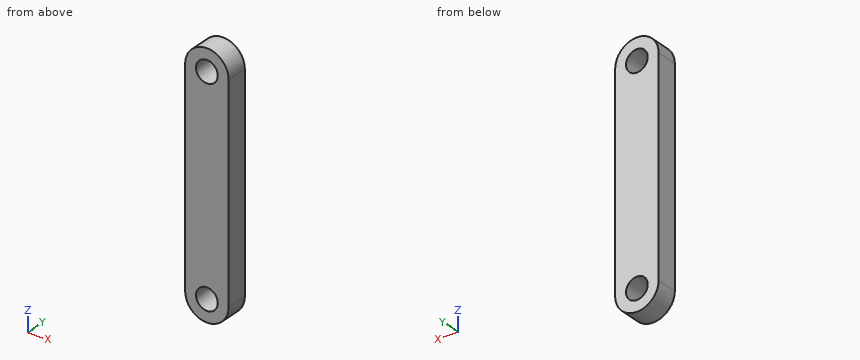
Autodesk Inventor part; units mm, degrees
ref_plane "YZ Plane" through (0, 0, 0) normal (1, 0, 0) x (0, 1, 0)
ref_plane "XZ Plane" through (0, 0, 0) normal (0, 1, 0) x (-1, 0, 0)
ref_plane "XY Plane" through (0, 0, 0) normal (0, 0, 1) x (1, 0, 0)
sketch "Boceto1" plane through (0, 0, 0) normal (0, 1, 0) x (-1, 0, 0)
  line L0 (0, -14.5) -> (0, 14.5) construction
  line L1 (3, -14.5) -> (3, 14.5)
  line L2 (-3, 14.5) -> (-3, -14.5)
  arc A0 (-3, -14.5) -> (3, -14.5) centre (0, -14.5) ccw
  arc A1 (3, 14.5) -> (-3, 14.5) centre (0, 14.5) ccw
  point P0 (0, 0)
  point P1 (0, 17.5)
  point P2 (0, -17.5)
  dimension "d0" = 14.5
  dimension "d1" = 6
extrude "Extrusión1" add sketch "Boceto1" along normal mid plane 3
sketch "Boceto2" plane through (0, 1.5, 0) normal (0, 1, 0) x (1, 0, 0)
  arc A0 (-3, -14.5) -> (3, -14.5) centre (0, -14.5) ccw construction
  arc A1 (3, 14.5) -> (-3, 14.5) centre (0, 14.5) ccw construction
  circle A2 centre (0, -14.5) radius 1.5
  circle A3 centre (0, 14.5) radius 1.5
  point P0 (0, 0)
  dimension "d4" = 3
  dimension "d5" = 3
extrude "Extrusión2" cut sketch "Boceto2" against normal blind 3
equation "\"Radio_pliegue\" = Grosor"
equation "\"Anchura_desahogo_plegado\" = Grosor"
equation "\"Profundidad_desahogo_plegado\" = 0.5 * Grosor"
equation "\"Tamaño_destalonado\" = 4 * Grosor"
equation "\"Remanente_mínimo\" = 2 * Grosor"
equation "\"Radiodetransición\" = Radio_pliegue"
equation "\"Tamaño_de_radio_de_Jacobi\" = Radio_pliegue"
equation "\"TamañoSeparación\" = Grosor"
properties part number "Pinza_pieza2"
Geometry: final body of the model. Coordinates: model frame, mm. Coordinates: 2 decimals unless noted, no trailing zeros. Order: outer loops, then holes, each group sorted by start corner. A loop starts at its lowest first (then second) coordinate and runs counter-clockwise, first axis right, second up. Notation, with made-up numbers: (56, -8.75) -> (94, -8.75) arc R21 cw to (94, -4.75) -> close; hole circle Ø5 at (21.5, 56.5). An arc over 180 degrees is marked (long way). Write each question's results on one line, items separated by ' | '. Start each with the question number.
1) Cut plane B-B, the plane y = 0.1. Output: boundary loops of the cut face in (x, z).
2) Cut plane C-C, the plane z = 15. Output: boundary loops of the cut face in (x, y), and give its area (3 significant figures).
3) Material intervals for line 1 along Z through (x, y) = (0, -0.8); line 2 along Z through (x, y) = (0.8, 0.1); line 3 along X through (y, z) = (0.25, 14.5), sorted ascending.
4) Cut plane A-A, the plane x = 0. Output: boundary loops of the cut face in (y, z).
5) Cut plane D-D, the plane x = 2.4. Output: boundary loops of the cut face in (y, z).
Checks:
1) outline: (-3, -14.5) arc R3 ccw to (3, -14.5) -> (3, 14.5) arc R3 ccw to (-3, 14.5) -> close; hole circle Ø3 at (0, -14.5); hole circle Ø3 at (0, 14.5)
2) outline: (-2.96, -1.5) -> (-1.41, -1.5) -> (-1.41, 1.5) -> (-2.96, 1.5) -> close; (1.41, -1.5) -> (2.96, -1.5) -> (2.96, 1.5) -> (1.41, 1.5) -> close | area: 9.26 mm^2
3) line 1: -17.5 to -16, -13 to 13, 16 to 17.5 | line 2: -17.39 to -15.77, -13.23 to 13.23, 15.77 to 17.39 | line 3: -3 to -1.5, 1.5 to 3
4) outline: (-1.5, -17.5) -> (1.5, -17.5) -> (1.5, -16) -> (-1.5, -16) -> close; (-1.5, -13) -> (1.5, -13) -> (1.5, 13) -> (-1.5, 13) -> close; (-1.5, 16) -> (1.5, 16) -> (1.5, 17.5) -> (-1.5, 17.5) -> close
5) outline: (-1.5, -16.3) -> (1.5, -16.3) -> (1.5, 16.3) -> (-1.5, 16.3) -> close
